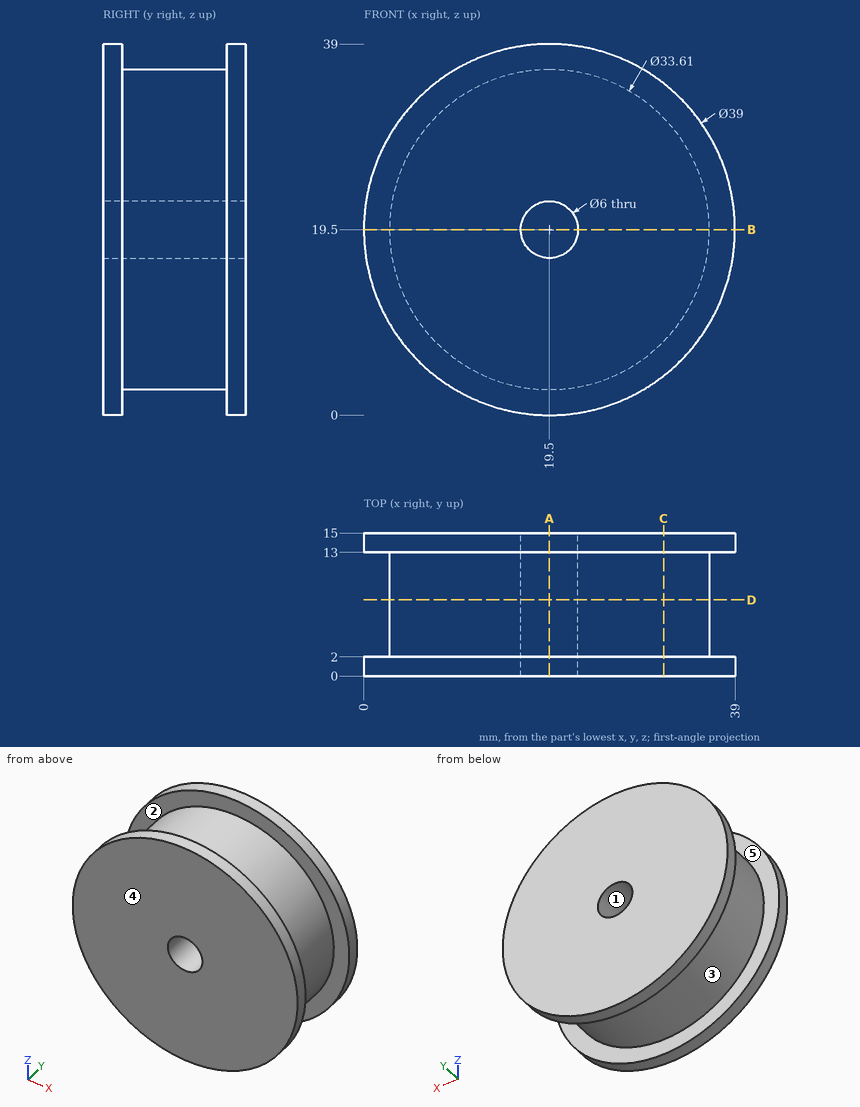
Answer from the drawing. Dimensions are ordinates in mm from the lowest x, y and z of the part. A direction names the side the tool comes from. Coordinates: 2 decimals unless noted, no trailing zeros. Write each loop counter-clockwise with the first axis right and the second up, starting at its lowest first coordinate (ties: lowest second). Pieces come first, ordered by that corner, then holes. Notation, with made-up numbers: (2, -8) - (41, -8) arc R10 cw to (41, -4) - close; hole circle Ø4 at (9.25, 58.5). An arc over 180 degrees is marked (long way). Return JSON: item names as keys, results as strings. Group by question number.
Q1. For a pull along X with two mould halves and no side action, classify the marked faces 1, 2 and 3 as +X half, -X half, draft (parallel to the pull), parting line (faces both ways), or undercut.
Q2. The part is cut by section C-C on x = 31.5. Write down the section's boundary in (y, z).
Q3. The part is cut by section B-B on z = 19.5. Write down the section's boundary in (x, y) (3 decimals), and give its area (3 significant figures).
Q4. Which of the six approach directions +Z, -Z, +X, -X, +Y, -Y give full straight-line access (tool end or side, diameter ignored) to the marked faces 4 and 5?
Q5. The part is cut by section A-A on x = 19.5. Write down the section's boundary in (y, z) (3 decimals), and give its area (3 significant figures).
Q6. Flat-ended cylindrical pins translate along their axes: pin 1 Ø4 at (y, z) = (6, 14) entering from -X; pin 2 Ø2 at (x, y) = (18.5, 4.5) entering from -Z (3 decimals). Find the tip coordinate at first contact, or state that the pin passes through.
Q7. Find the intervals of material crossed by line 1 along Y through (x, z) = (8.5, 34); line 2 along X through (y, z) = (5.75, 19.5) (3 decimals); line 3 along X through (y, z) = (4, 17.5), in increasing order. Write a range as [from, to].
Q8. The part is cut by section D-D on y = 8. Write down the section's boundary in (x, z) (3 decimals).
Evaluation:
{
 "1": {"face 1": "undercut", "face 2": "draft", "face 3": "parting line"},
 "2": {"outline": "(0, 4.13) - (2, 4.13) - (2, 7.74) - (13, 7.74) - (13, 4.13) - (15, 4.13) - (15, 34.87) - (13, 34.87) - (13, 31.26) - (2, 31.26) - (2, 34.87) - (0, 34.87) - close"},
 "3": {"outline": "(0, 0) - (16.5, 0) - (16.5, 15) - (0, 15) - (0, 13) - (2.695, 13) - (2.695, 2) - (0, 2) - close; (22.5, 0) - (39, 0) - (39, 2) - (36.305, 2) - (36.305, 13) - (39, 13) - (39, 15) - (22.5, 15) - close", "area": "436 mm2"},
 "4": {"face 4": "+Z, -Z, +X, -X, -Y", "face 5": "none"},
 "5": {"outline": "(0, 0) - (2, 0) - (2, 2.695) - (13, 2.695) - (13, 0) - (15, 0) - (15, 16.5) - (0, 16.5) - close; (0, 22.5) - (15, 22.5) - (15, 39) - (13, 39) - (13, 36.305) - (2, 36.305) - (2, 39) - (0, 39) - close", "area": "436 mm2"},
 "6": {"pin 1": "stops at x = 3.06", "pin 2": "stops at z = 2.695"},
 "7": {"line 1": "y = [0, 2], [13, 15]", "line 2": "x = [2.695, 16.5], [22.5, 36.305]", "line 3": "x = [2.81, 17.26], [21.74, 36.19]"},
 "8": {"outline": "circle Ø33.61 at (19.5, 19.5); hole circle Ø6 at (19.5, 19.5)"}
}
